The listing builds one solid part. Answer for the finished solid, in the listing's coordinates (mm). Round coordinates to 2 decimals unless told otherwise and drop trailing zeros. Write each loop counter-clockwise with the first axis right and the second up, starting at its lowest first coordinate (ties: lowest second). Pieces come first, ordered by that corner, then holes.
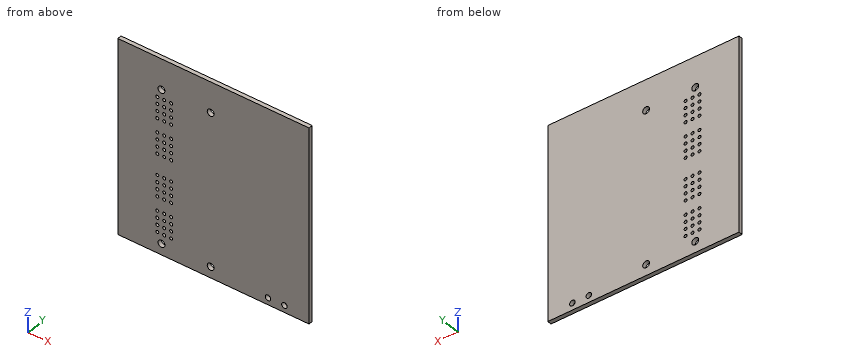
from build123d import *

# Parameters (mm, degrees)
ESBO_O1_W                = 70
ESBO_O1_H                = 70
ESBO_O1_R                = 1.25
ESBO_O1_R_2              = 1
RESSALTO_EXTRUS_O1_DEPTH = 1.5
ESBO_O2_R                = 0.55
CORTE_EXTRUS_O1_DEPTH    = 50.520197899
PADR_O_LINEAR1_COUNT     = 20
PADR_O_LINEAR1_PITCH     = 2.54


with BuildPart() as part:
    # Esboço1 → Ressalto-extrusão1 (new body)
    with BuildSketch(Plane(origin=(0, 0, 0), x_dir=(1, 0, 0), z_dir=(0, 1, 0))):
        Rectangle(ESBO_O1_W, ESBO_O1_H)
        with Locations(Location((-19, 31, 0), (0, 0, 270))):
            Circle(ESBO_O1_R, mode=Mode.SUBTRACT)
        with Locations(Location((-1, 31, 0), (0, 0, 270))):
            Circle(ESBO_O1_R, mode=Mode.SUBTRACT)
        with Locations(Location((-1, -24, 0), (0, 0, 270))):
            Circle(ESBO_O1_R, mode=Mode.SUBTRACT)
        with Locations(Location((-19, -24, 0), (0, 0, 270))):
            Circle(ESBO_O1_R, mode=Mode.SUBTRACT)
        with Locations(Location((20, 32.5, 0), (0, 0, 270))):
            Circle(ESBO_O1_R_2, mode=Mode.SUBTRACT)
        with Locations(Location((26, 32.5, 0), (0, 0, 270))):
            Circle(ESBO_O1_R_2, mode=Mode.SUBTRACT)
    extrude(amount=RESSALTO_EXTRUS_O1_DEPTH)

    # Esboço2 → Corte-extrusão1 (cut, through all)
    with BuildSketch(Plane(origin=(0, 1.5, 0), x_dir=(1, 0, 0), z_dir=(0, 1, 0))):
        with Locations(Location((-20.54, 27.5, 0), (0, 0, 270))):
            Circle(ESBO_O2_R)
        with Locations(Location((-18, 27.5, 0), (0, 0, 270))):
            Circle(ESBO_O2_R)
        with Locations(Location((-15.46, 27.5, 0), (0, 0, 270))):
            Circle(ESBO_O2_R)
    corte_extrus_o1 = extrude(amount=-CORTE_EXTRUS_O1_DEPTH, mode=Mode.SUBTRACT)

    # Padrão linear1: Corte-extrusão1 ×20, 4 skipped
    with Locations(*[(0, 0, i * PADR_O_LINEAR1_PITCH) for i in range(1, PADR_O_LINEAR1_COUNT) if i not in (4, 9, 10, 15)]):
        add(corte_extrus_o1, mode=Mode.SUBTRACT)


solid = part.part
1. Straight lines are drawn through the part: line 1 along X through (y, z) = (0.85, 8.06); line 2 along Z through (x, y) = (-1.5, 1.05); line 3 along Z through (x, y) = (-2, 0.15). For each, find the intervals that lie inside material, in ascending order.
Geometry says:
line 1: x = -35 to -21.09, -19.99 to -18.55, -17.45 to -16.01, -14.91 to 35
line 2: z = -35 to -32.15, -29.85 to 22.85, 25.15 to 35
line 3: z = -35 to -31.75, -30.25 to 23.25, 24.75 to 35
2. Given pin 1 (1.3 mm diameter, centred on x = -18, z = 5.52, fed in from -Y), flat-ended and moving along its own axis, determine where the tip first touches the part or whether it passes through.
Geometry says:
pin 1: stops at y = 0
3. Section A-A on z = 24 is taken. Determine the outline of the cut face in (x, y), plus the area to 3 significant figures.
Geometry says:
outline: (-35, 0) - (-20.25, 0) - (-20.25, 1.5) - (-35, 1.5) - close; (-17.75, 0) - (-2.25, 0) - (-2.25, 1.5) - (-17.75, 1.5) - close; (0.25, 0) - (35, 0) - (35, 1.5) - (0.25, 1.5) - close
area: 97.5 mm2
